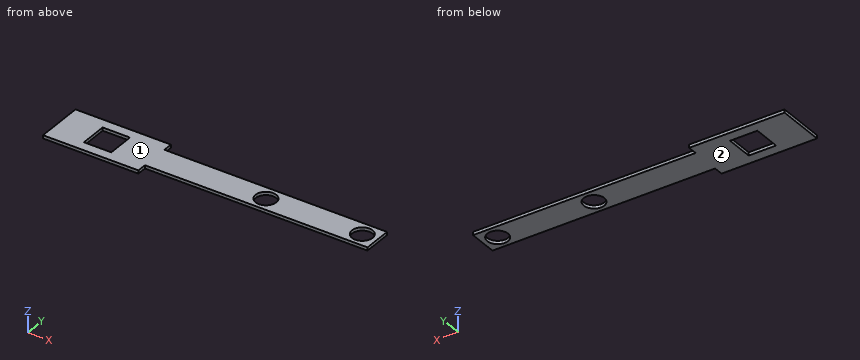
from build123d import *

# Parameters (mm, degrees)
BOSS_EXTRUDE1_DEPTH     = 1
SKETCH3_W               = 8.6
SKETCH3_H               = 8.6
CUT_EXTRUDE2_DEPTH      = 102.123686642
CUT_EXTRUDE3_DEPTH      = 102.123686642
CUT_EXTRUDE3_DEPTH_BACK = 102.123686642
SKETCH5_R               = 3.25


with BuildPart() as part:
    # Sketch1 → Boss-Extrude1 (new body)
    with BuildSketch(Plane.XY):
        Polygon((30, -3), (30, 0), (0, 0), (0, -15), (30, -15), (30, -12), (100, -12), (100, -3), align=None)
    extrude(amount=BOSS_EXTRUDE1_DEPTH)

    # Sketch3 → Cut-Extrude2 (cut, through all)
    with BuildSketch(Plane(origin=(0, 0, 0), x_dir=(-1, 0, 0), z_dir=(0, 0, -1))):
        with Locations((-15, -7.5)):
            Rectangle(SKETCH3_W, SKETCH3_H)
    extrude(amount=-CUT_EXTRUDE2_DEPTH, mode=Mode.SUBTRACT)

    # Sketch5 → Cut-Extrude3 (cut, two sides: drawn at the far end of the back side and taken through both)
    with BuildSketch(Plane.XY.offset(1).offset(-CUT_EXTRUDE3_DEPTH_BACK)):
        with Locations((65, -7.5)):
            Circle(SKETCH5_R)
        with Locations((95.3, -7.5)):
            Circle(SKETCH5_R)
    extrude(amount=CUT_EXTRUDE3_DEPTH + CUT_EXTRUDE3_DEPTH_BACK, mode=Mode.SUBTRACT)


solid = part.part
Verification items for the finished model (mm, model axes). Face numbers are marked on the shaded views. Coordinates: 2 decimals unless noted, no trailing zeros. Order: outer loops, then holes, each group sorted by start corner. A loop starts at its lowest first (then second) coordinate and runs counter-clockwise, first axis right, second up.
Item 1: Material ranges on L1, parallel to X at y = -7.5, z = 0.8; L2, parallel to Y at x = 65, z = 0.6; L3, parallel to X at y = -2.75, z = 0.2, recorded low to high.
Filled in:
L1: x = 0 to 10.7, 19.3 to 61.75, 68.25 to 92.05, 98.55 to 100
L2: y = -12 to -10.75, -4.25 to -3
L3: x = 0 to 30
Item 2: Section check D-D, the plane x = 33. Enter the section's corners in (y, z), then the cut area to 3 significant figures.
Filled in:
outline: (-12, 0) - (-3, 0) - (-3, 1) - (-12, 1) - close
area: 9.00 mm2
Item 3: Depth check by flat-ended pin: pin 1 (8.5 mm diameter, centred on x = 65, y = -7.5, fed in from -Z). Enter the tip coordinate at first touch or a pass-through.
Filled in:
pin 1: stops at z = 0
Item 4: Release check for a two-part mould opening along Z. For the marked faces 1 and 2 record: +Z half, -Z half, draft (parallel to the pull), parting line (faces both ways), or undercut.
Filled in:
face 1: +Z half
face 2: -Z half
Item 5: Section check A-A, the plane y = -7.5. Enter the section's corners in (x, z).
Filled in:
outline: (0, 0) - (10.7, 0) - (10.7, 1) - (0, 1) - close; (19.3, 0) - (61.75, 0) - (61.75, 1) - (19.3, 1) - close; (68.25, 0) - (92.05, 0) - (92.05, 1) - (68.25, 1) - close; (98.55, 0) - (100, 0) - (100, 1) - (98.55, 1) - close
Item 6: Section check C-C, the plane z = 0.4. Enter the section's corners in (x, y).
Filled in:
outline: (0, -15) - (30, -15) - (30, -12) - (100, -12) - (100, -3) - (30, -3) - (30, 0) - (0, 0) - close; hole (10.7, -11.8) - (19.3, -11.8) - (19.3, -3.2) - (10.7, -3.2) - close; hole circle Ø6.5 at (65, -7.5); hole circle Ø6.5 at (95.3, -7.5)
Item 7: Section check B-B, the plane x = 95.3. Enter the section's corners in (y, z).
Filled in:
outline: (-12, 0) - (-10.75, 0) - (-10.75, 1) - (-12, 1) - close; (-4.25, 0) - (-3, 0) - (-3, 1) - (-4.25, 1) - close
